Here's how the part is built. I have some questions about the finished solid (model axes, mm). A direction names the side the tool comes from. Give positions to 0.01 mm unless a question says otherwise; leave off trailing zeros. Order: outer loops, then holes, each group sorted by start corner. A loop starts at its lowest first (then second) coordinate and runs counter-clockwise, first axis right, second up. Notation, with made-up numbers: M 87,77.25 L 131,77.25 A18 cw 131,108.25 Z; hole C 53,-26.5 d8. An arc over 180 degrees is marked long. Use one line per item in the form item = value.
from build123d import *

# Parameters (mm, degrees)
SKETCH_1_R               = 1.5
SKETCH_1_W               = 4
SKETCH_1_H               = 11.3
EXTRUDE_1_DEPTH          = 1
SKETCH_2_W               = 2.5
SKETCH_2_H               = 11.3
EXTRUDE_2_DEPTH          = 22
SKETCH_3_W               = 40.1
SKETCH_3_H               = 11.3
EXTRUDE_3_DEPTH          = 2
SKETCH_4_R               = 10
EXTRUDE_4_DEPTH          = 2
EXTRUDE_START            = 30
SKETCH_6_R               = 10
EXTRUDE_5_DEPTH          = 30
CUT_EXTRUDE_2_DEPTH      = 60.690242084
CUT_EXTRUDE_2_DEPTH_BACK = 60.690242084
SKETCH_8_R               = 2.5
CUT_EXTRUDE_3_DEPTH      = 69.000073623
CUT_EXTRUDE_3_DEPTH_BACK = 69.000073623
SKETCH_9_R               = 2.5


with BuildPart() as part:
    # 草图1 → 凸台-拉伸1 (new body)
    # profile 1 of 4: a face of its own
    with BuildSketch(Plane.XY):
        Polygon((-12.05, -5.65), (-12.05, 0), (-12.05, 5.65), (-16.05, 5.65), (-16.05, -5.65), align=None)
        with Locations((-13.65, 0)):
            Circle(SKETCH_1_R, mode=Mode.SUBTRACT)
    # profile 2 of 4: a face of its own
    with BuildSketch(Plane.XY):
        Polygon((12.05, 5.65), (12.05, 0), (12.05, -5.65), (16.05, -5.65), (16.05, 5.65), align=None)
        with BuildLine():
            ThreePointArc((15.15, 0), (13.65, -1.5), (12.15, 0))
            ThreePointArc((12.15, 0), (13.65, 1.5), (15.15, 0))
        make_face(mode=Mode.SUBTRACT)
    # profile 3 of 4: a face of its own
    with BuildSketch(Plane.XY):
        with Locations((-18.05, 0)):
            Rectangle(SKETCH_1_W, SKETCH_1_H)
    # profile 4 of 4: a face of its own
    with BuildSketch(Plane.XY):
        with Locations((18.05, 0)):
            Rectangle(SKETCH_1_W, SKETCH_1_H)
    extrude(amount=-EXTRUDE_1_DEPTH)

    # 草图2 → 凸台-拉伸2 (add)
    with BuildSketch(Plane.XY):
        with Locations((-18.8, 0)):
            Rectangle(SKETCH_2_W, SKETCH_2_H)
        with Locations((18.8, 0)):
            Rectangle(SKETCH_2_W, SKETCH_2_H)
    extrude(amount=EXTRUDE_2_DEPTH)

    # 草图3 → 凸台-拉伸3 (add)
    with BuildSketch(Plane.XY.offset(22)):
        Rectangle(SKETCH_3_W, SKETCH_3_H)
    extrude(amount=EXTRUDE_3_DEPTH)

    # 草图4 → 凸台-拉伸4 (add)
    with BuildSketch(Plane.XY.offset(24)):
        Circle(SKETCH_4_R)
    extrude(amount=-EXTRUDE_4_DEPTH)

    # 草图6 → 凸台-拉伸5 (add)
    with BuildSketch(Plane.XY.offset(24).offset(EXTRUDE_START)):
        Circle(SKETCH_6_R)
    extrude(amount=-EXTRUDE_5_DEPTH)

    # 草图8 → 切除-拉伸2 (cut, two sides: drawn at the far end of the back side and taken through both)
    with BuildSketch(Plane.XZ.offset(5.65).offset(-CUT_EXTRUDE_2_DEPTH_BACK)):
        with Locations(Location((0, 46.5, 0), (0, 0, 270))):
            Circle(SKETCH_8_R)
    extrude(amount=CUT_EXTRUDE_2_DEPTH + CUT_EXTRUDE_2_DEPTH_BACK, mode=Mode.SUBTRACT)

    # 草图9 → 切除-拉伸3 (cut, two sides: drawn at the far end of the back side and taken through both)
    with BuildSketch(Plane.ZY.offset(20.05).offset(-CUT_EXTRUDE_3_DEPTH_BACK)):
        with Locations(Location((36.5, 0, 0), (0, 0, 270))):
            Circle(SKETCH_9_R)
    extrude(amount=CUT_EXTRUDE_3_DEPTH + CUT_EXTRUDE_3_DEPTH_BACK, mode=Mode.SUBTRACT)


solid = part.part
Q1. Thinking about a two-plate mould opening in X: for faces 4 (the face through (20.05, 0, 11)), 5 (the face through (16, 0, -1)), 6 (the face through (-0.96, 0.14, 44.19)), which applies, +X half, -X half, draft (parallel to the pull), parting line (faces both ways), or undercut?
Found:
face_4 = +X half
face_5 = draft
face_6 = undercut
Q2. On a 3-axis mill with a long thin cutter (end or side, diameter ignored), from which of +Z, -Z, +X, -X, +Y, -Y can I reach the whole of each face in a straight line? I mean faces 1 (the face through (-17.55, 0, 11)), 2 (the face through (-15.15, 0.07, -0.49)), 3 (the face through (-18, 5.65, 12)). Say none if no direction works.
Found:
face_1 = +Y, -Y
face_2 = -Z
face_3 = +Z, -Z, -X, +Y
Q3. I'm going to push flat-ended pins straight in: pin 1 Ø10 at (y, z) = (-7.5, 40) entering from +X; pin 2 Ø3.5 at (x, y) = (12, -0.5) entering from +Z; pin 3 Ø6.5 at (y, z) = (0, 36.5) entering from -X. Where does each tip first touch, or does it pass through?
Found:
pin_1 = 9.68
pin_2 = 24
pin_3 = -10
Q4. I need wall thicknesses on L1, parallel to Z at x = 0, y = 2.75; L2, parallel to Z at x = -17.5, y = 2.75; L3, parallel to X at y = 1, z = 16.5. Which ranges of each line are inside material? Lowest first, please.
Found:
L1 = 22 to 44, 49 to 54
L2 = -1 to 0, 22 to 24
L3 = -20.05 to -17.55, 17.55 to 20.05
Q5. I want a section at D-D on z = 11. Write out the boundary of the cut face in (x, y), then the cut area to 3 significant figures.
Found:
outline = M -20.05,-5.65 L -17.55,-5.65 L -17.55,5.65 L -20.05,5.65 Z; M 17.55,-5.65 L 20.05,-5.65 L 20.05,5.65 L 17.55,5.65 Z
area = 56.5 mm²
Q6. I want a section at A-A on x = 0. Write out the boundary of the cut face in (y, z).
Found:
outline = M -10,22 L 10,22 L 10,44 L -10,44 Z; M -10,49 L 10,49 L 10,54 L -10,54 Z; hole C 0,36.5 d5
Q7. I want a section at B-B on y = 0. State how many separate pieces and enclosed holes the cut face has, then the cut area to 3 significant figures.
Found:
separate_pieces = 4
enclosed_holes = 1
area = 681 mm²
Q8. I want a section at C-C on x = 13.65. Write out the boundary of the cut face in (y, z).
Found:
outline = M -5.65,-1 L -1.5,-1 L -1.5,0 L -5.65,0 Z; M -5.65,22 L 5.65,22 L 5.65,24 L -5.65,24 Z; M 1.5,-1 L 5.65,-1 L 5.65,0 L 1.5,0 Z
